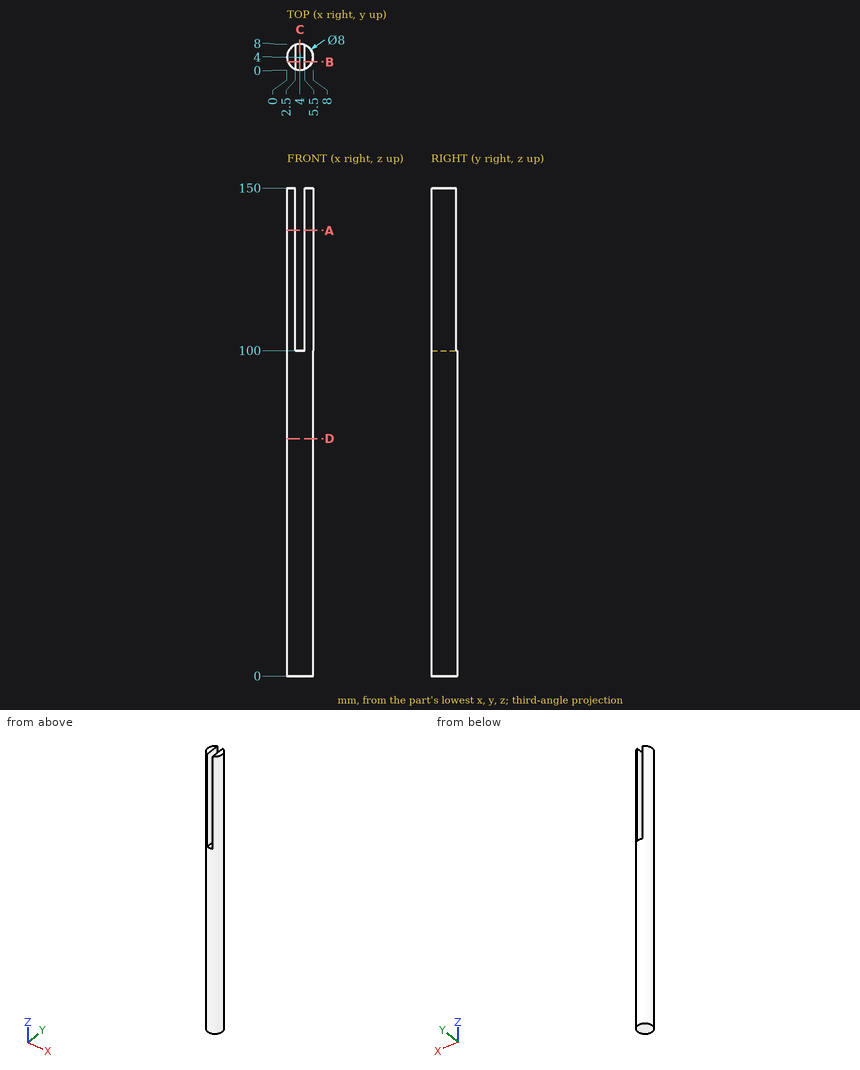
Print and shaded views of the part. All mm, measured from the part's lowest x, y and z. Coordinates: 2 decimals unless noted, no trailing zeros. Write each loop counter-clockwise with the first axis right and the second up, starting at its lowest first coordinate (ties: lowest second). Pieces come first, ordered by that corner, then holes. Notation, with made-up numbers: (32.5, 4.5) - (52.5, 4.5) arc R12 cw to (52.5, 23.5) - close; hole circle Ø6 at (15.5, 2.5). An arc over 180 degrees is marked (long way). One line per question, with ' | ' between items. Start each with the question number.
Q1. Drill centre lines: line 1 (Z direction, x = 3.25, y = 2.5); line 2 (X direction, y = 5.75, z = 130); line 3 (X direction, y = 3, z = 116). Where is each one in solid material? Low to high. Write a range as [from, to].
Q2. Pin check, flat tips, straight feed: pin 1 (2 mm diameter, centred on y = 6, z = 123, fed in from +X); pin 2 (2 mm diameter, centred on y = 7, z = 27.5, fed in from -X). Stop position of each tip, or through.
Q3. Cut at B-B, the plane y = 2.5. List the corners of the cut face in (x, z).
Q4. Cut at C-C, the plane x = 4. List the corners of the cut face in (y, z), then the cut area to 3 significant figures.
Q5. Cut at D-D, the plane z = 73. List the corners of the cut face in (x, y), then the cut area to 3 significant figures.
Q6. Cut at A-A, the plane z = 137. List the corners of the cut face in (x, y), then the cut area to 3 significant figures.
Answer below:
1) line 1: [0, 100] | line 2: [0.4, 2.5], [5.5, 7.6] | line 3: [0.13, 2.5], [5.5, 7.87]
2) pin 1: x = 7.87 | pin 2: x = 0.54
3) outline: (0.29, 0) - (7.71, 0) - (7.71, 150) - (5.5, 150) - (5.5, 100) - (2.5, 100) - (2.5, 150) - (0.29, 150) - close
4) outline: (0, 0) - (8, 0) - (8, 100) - (0, 100) - close | area: 800 mm^2
5) outline: circle Ø8 at (4, 4) | area: 50.3 mm^2
6) outline: (2.5, 0.29) - (2.5, 7.71) arc R4 ccw to start; (5.5, 0.29) arc R4 ccw to (5.5, 7.71) - close | area: 26.8 mm^2
